The listing builds one solid part. Answer for the finished solid, in the listing's coordinates (mm). Coordinates: 2 decimals unless noted, no trailing zeros. Loops run counter-clockwise (first coordinate to the right, second up) from the corner with the lowest first, then second, coordinate; pieces in that order, holes last. Notation, with made-up numbers: (-32, 83) -> (-10, 83) arc R25 cw to (-10, 95) -> close; hole circle Ø7 at (-10.5, 29). An arc over 180 degrees is marked (long way). Answer in a Markdown table with one row per item.
```python
from build123d import *

# Parameters (mm, degrees)
EXTRUDE_1_DEPTH     = 4
SKETCH_2_R          = 1.5
CUT_EXTRUDE_1_DEPTH = 184.032783949


with BuildPart() as part:
    # 草图1 → 凸台-拉伸1 (new body)
    with BuildSketch(Plane(origin=(0, 0, 0), x_dir=(1, 0, 0), z_dir=(0, 1, 0))):
        with BuildLine():
            Line((-119.819061856, 72.980279065), (-162.812846416, 32.966261751))
            ThreePointArc((-162.812846416, 32.966261751), (-165.168654868, 29.638038623), (-166, 25.646075708))
            Line((-166, 25.646075708), (-166, -25.646075708))
            ThreePointArc((-166, -25.646075708), (-165.168654868, -29.638038623), (-162.812846416, -32.966261751))
            Line((-162.812846416, -32.966261751), (-119.819061856, -72.980279065))
            ThreePointArc((-119.819061856, -72.980279065), (-115.090503207, -75.958943119), (-109.599792231, -77))
            Line((-109.599792231, -77), (109.599792231, -77))
            ThreePointArc((109.599792231, -77), (115.090503207, -75.958943119), (119.819061856, -72.980279065))
            Line((119.819061856, -72.980279065), (162.812846416, -32.966261751))
            ThreePointArc((162.812846416, -32.966261751), (165.168654868, -29.638038623), (166, -25.646075708))
            Line((166, -25.646075708), (166, 25.646075708))
            ThreePointArc((166, 25.646075708), (165.168654868, 29.638038623), (162.812846416, 32.966261751))
            Line((162.812846416, 32.966261751), (119.819061856, 72.980279065))
            ThreePointArc((119.819061856, 72.980279065), (115.090503207, 75.958943119), (109.599792231, 77))
            Line((109.599792231, 77), (-109.599792231, 77))
            ThreePointArc((-109.599792231, 77), (-115.090503207, 75.958943119), (-119.819061856, 72.980279065))
        make_face()
    extrude(amount=EXTRUDE_1_DEPTH)

    # 草图2 → 切除-拉伸1 (cut, through all)
    with BuildSketch(Plane.XZ):
        with Locations(Location((5, 25, 0), (0, 0, 270))):
            Circle(SKETCH_2_R)
        with Locations(Location((-5, 25, 0), (0, 0, 270))):
            Circle(SKETCH_2_R)
        with Locations(Location((-5, 15, 0), (0, 0, 270))):
            Circle(SKETCH_2_R)
        with Locations(Location((5, 15, 0), (0, 0, 270))):
            Circle(SKETCH_2_R)
        with Locations(Location((-5, -15, 0), (0, 0, 270))):
            Circle(SKETCH_2_R)
        with Locations(Location((5, -15, 0), (0, 0, 270))):
            Circle(SKETCH_2_R)
        with Locations(Location((-5, -25, 0), (0, 0, 270))):
            Circle(SKETCH_2_R)
        with Locations(Location((5, -25, 0), (0, 0, 270))):
            Circle(SKETCH_2_R)
        with Locations(Location((-70.7, -15, 0), (0, 0, 270))):
            Circle(SKETCH_2_R)
        with Locations(Location((-70.7, -25, 0), (0, 0, 270))):
            Circle(SKETCH_2_R)
        with Locations(Location((-80.7, -25, 0), (0, 0, 270))):
            Circle(SKETCH_2_R)
        with Locations(Location((-80.7, -15, 0), (0, 0, 270))):
            Circle(SKETCH_2_R)
        with Locations(Location((-70.7, 25, 0), (0, 0, 270))):
            Circle(SKETCH_2_R)
        with Locations(Location((-80.7, 25, 0), (0, 0, 270))):
            Circle(SKETCH_2_R)
        with Locations(Location((-80.7, 15, 0), (0, 0, 270))):
            Circle(SKETCH_2_R)
        with Locations(Location((-70.7, 15, 0), (0, 0, 270))):
            Circle(SKETCH_2_R)
        with Locations(Location((70.7, 25, 0), (0, 0, 270))):
            Circle(SKETCH_2_R)
        with Locations(Location((70.7, 15, 0), (0, 0, 270))):
            Circle(SKETCH_2_R)
        with Locations(Location((80.7, 15, 0), (0, 0, 270))):
            Circle(SKETCH_2_R)
        with Locations(Location((80.7, 25, 0), (0, 0, 270))):
            Circle(SKETCH_2_R)
        with Locations(Location((70.7, -15, 0), (0, 0, 270))):
            Circle(SKETCH_2_R)
        with Locations(Location((80.7, -15, 0), (0, 0, 270))):
            Circle(SKETCH_2_R)
        with Locations(Location((70.7, -25, 0), (0, 0, 270))):
            Circle(SKETCH_2_R)
        with Locations(Location((80.7, -25, 0), (0, 0, 270))):
            Circle(SKETCH_2_R)
        with Locations(Location((5, -72, 0), (0, 0, 270))):
            Circle(SKETCH_2_R)
        with Locations(Location((-5, -72, 0), (0, 0, 270))):
            Circle(SKETCH_2_R)
        with Locations(Location((-5, 72, 0), (0, 0, 90))):
            Circle(SKETCH_2_R)
        with Locations(Location((5, 72, 0), (0, 0, 90))):
            Circle(SKETCH_2_R)
        with Locations(Location((-145, 20, 0), (0, 0, 270))):
            Circle(SKETCH_2_R)
        with Locations(Location((-135, 20, 0), (0, 0, 270))):
            Circle(SKETCH_2_R)
        with Locations(Location((-145, -20, 0), (0, 0, 270))):
            Circle(SKETCH_2_R)
        with Locations(Location((-135, -20, 0), (0, 0, 270))):
            Circle(SKETCH_2_R)
        with Locations(Location((145, 20, 0), (0, 0, 90))):
            Circle(SKETCH_2_R)
        with Locations(Location((135, -20, 0), (0, 0, 90))):
            Circle(SKETCH_2_R)
        with Locations(Location((135, 20, 0), (0, 0, 90))):
            Circle(SKETCH_2_R)
        with Locations(Location((145, -20, 0), (0, 0, 90))):
            Circle(SKETCH_2_R)
    extrude(amount=-CUT_EXTRUDE_1_DEPTH, mode=Mode.SUBTRACT)


solid = part.part
```
Item 1: Flat-ended cylindrical pins translate along their axes: pin 1 Ø1.5 at (x, y) = (-129.5, 1.5) entering from -Z; pin 2 Ø1 at (y, z) = (1, -53.5) entering from -X; pin 3 Ø2.5 at (x, z) = (80.7, 15) entering from -Y. Find the tip coordinate at first contact, or state that the pin passes through.
Findings below:
| item | result |
|---|---|
| pin 1 | stops at z = -64.67 |
| pin 2 | stops at x = -141.29 |
| pin 3 | passes through |
Item 2: A cutting plane is placed at C-C, the plane z = -46. Determine the outline of the cut face in (x, y).
Findings below:
| item | result |
|---|---|
| outline | (-148.81, 0) -> (148.81, 0) -> (148.81, 4) -> (-148.81, 4) -> close |
Item 3: Find the intervals of material crossed by probe 1 along Z at (x, y) = (-70.7, 3.15); probe 2 along Z at (x, y) = (145, 2.6); probe 3 along X at (y, z) = (2.75, -20), in increasing order.
Findings below:
| item | result |
|---|---|
| probe 1 | z = -77 to -26.5, -23.5 to -16.5, -13.5 to 13.5, 16.5 to 23.5, 26.5 to 77 |
| probe 2 | z = -49.54 to -21.5, -18.5 to 18.5, 21.5 to 49.54 |
| probe 3 | x = -166 to -146.5, -143.5 to -136.5, -133.5 to 133.5, 136.5 to 143.5, 146.5 to 166 |
Item 4: A cutting plane is placed at A-A, the plane y = 2.2. Count the separate pieces of the cut face and the enclosed holes in it, plus the area to 3 significant figures.
Findings below:
| item | result |
|---|---|
| separate pieces | 1 |
| enclosed holes | 36 |
| area | 46,100 mm2 |
Item 5: A cutting plane is placed at B-B, the plane z = 60. Determine the outline of the cut face in (x, y).
Findings below:
| item | result |
|---|---|
| outline | (-133.77, 0) -> (133.77, 0) -> (133.77, 4) -> (-133.77, 4) -> close |
